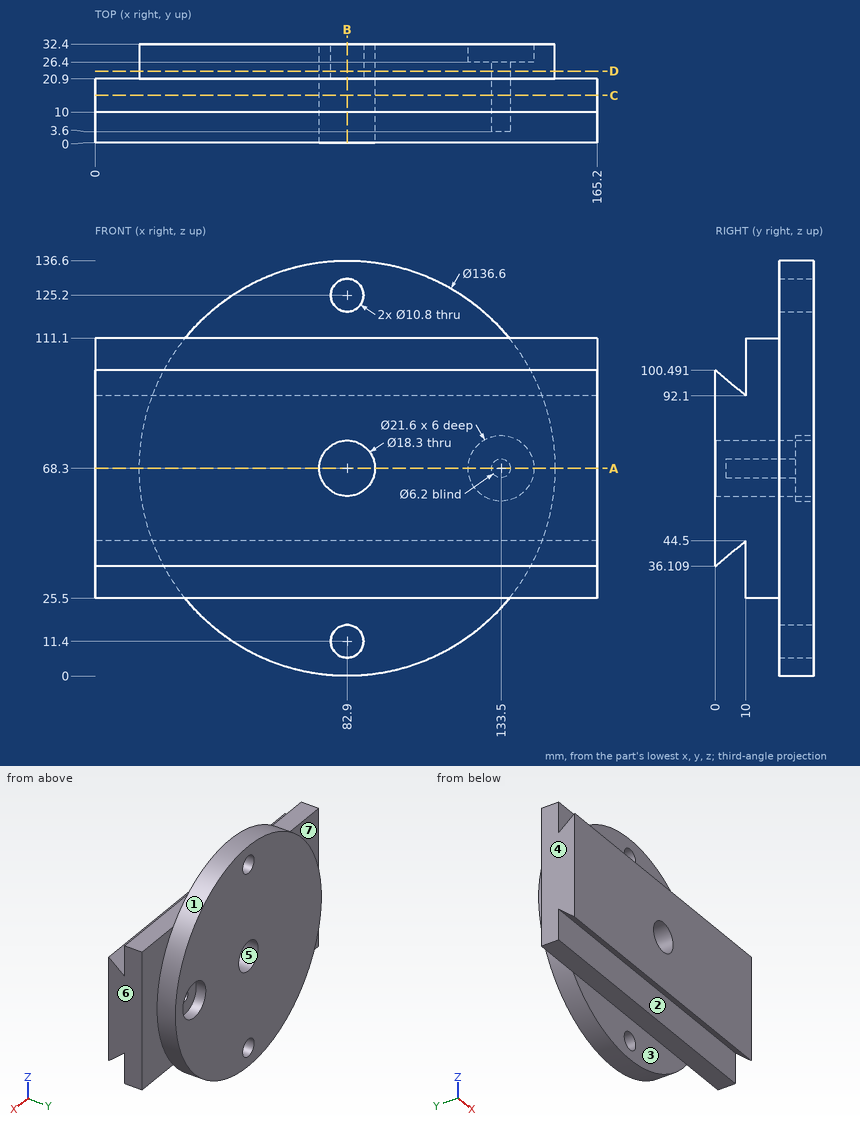
Design review of the part shown in the three views and the two pictorial views. Dimensions are in mm from the part's minimum x, y and z. A direction names the side the tool comes from. Give positions to 0.01 mm unless a question says otherwise; leave off trailing zeros. Write each loop counter-clockwise with the first axis right and the second up, starting at its lowest first coordinate (ties: lowest second). Pieces come first, ordered by that corner, then holes.
Item 1: Take a section at D-D (y = 23.5). Give the boundary of the cut face in (x, z), and give its area (3 significant figures).
Item 2: Take a section at B-B (x = 82.9). Give the boundary of the cut face in (y, z), and give its area (3 significant figures).
Item 3: Machinability: for the marked faces 1, 2 and 3, which of the approach directions +Z, -Z, +X, -X, +Y, -Y give a long, thin tool a straight path to every point of the face, cutting with its end or side? Answer none if there is none.
Item 4: Wall thickness on probe 1 along X at (y, z) = (30, 68); probe 2 along Z at (x, y) = (82.9, 28); probe 3 along Z at (x, y) = (133.5, 16.5): over which ranges is each line inside the solid? List them lowest first.
Item 5: Take a section at A-A (z = 68.3). Give the boundary of the cut face in (x, y), and give its area (3 significant figures).
Item 6: Take a section at C-C (y = 15.5). Give the boundary of the cut face in (x, z).
Item 7: Insertion check: P1, Ø20.5, axis at x = 105, z = 18, coming from the -Y side; P2, Ø1, axis at x = 50, y = 12, coming from the +Z side; P3, Ø3, axis at x = 134, z = 67.5, coming from the +Y side. Each pin has a flat end and moves straight along its axis. Give the tip position at first contact, or say it passes through.
Item 8: The part is to be moulded in two halves that separate along X. For the marked faces 4, 5, 6 and 7, say which applies: +X half, -X half, draft (parallel to the pull), parting line (faces both ways), or undercut.
Established:
1. outline: circle Ø136.6 at (82.9, 68.3); hole circle Ø18.3 at (82.9, 68.3); hole circle Ø10.8 at (82.9, 11.4); hole circle Ø10.8 at (82.9, 125.2); hole circle Ø6.2 at (133.5, 68.3)
1. area: 14,200 mm2
2. outline: (0, 36.11) - (10, 44.5) - (10, 25.5) - (20.9, 25.5) - (20.9, 16.8) - (32.4, 16.8) - (32.4, 59.15) - (0, 59.15) - close; (0, 77.45) - (32.4, 77.45) - (32.4, 119.8) - (20.9, 119.8) - (20.9, 111.1) - (10, 111.1) - (10, 92.1) - (0, 100.49) - close; (20.9, 0) - (32.4, 0) - (32.4, 6) - (20.9, 6) - close; (20.9, 130.6) - (32.4, 130.6) - (32.4, 136.6) - (20.9, 136.6) - close
2. area: 2,220 mm2
3. face 1: +Y
3. face 2: -Z, +X, -X
3. face 3: -Z, +X, -X, -Y
4. probe 1: x = 14.6 to 73.75, 92.05 to 122.7, 144.3 to 151.2
4. probe 2: z = 0 to 6, 16.8 to 59.15, 77.45 to 119.8, 130.6 to 136.6
4. probe 3: z = 25.5 to 65.2, 71.4 to 111.1
5. outline: (0, 0) - (73.75, 0) - (73.75, 32.4) - (14.6, 32.4) - (14.6, 20.9) - (0, 20.9) - close; (92.05, 0) - (165.2, 0) - (165.2, 20.9) - (151.2, 20.9) - (151.2, 32.4) - (144.3, 32.4) - (144.3, 26.4) - (136.6, 26.4) - (136.6, 3.6) - (130.4, 3.6) - (130.4, 26.4) - (122.7, 26.4) - (122.7, 32.4) - (92.05, 32.4) - close
5. area: 4,160 mm2
6. outline: (0, 25.5) - (165.2, 25.5) - (165.2, 111.1) - (0, 111.1) - close; hole circle Ø18.3 at (82.9, 68.3); hole circle Ø6.2 at (133.5, 68.3)
7. P1: stops at y = 10
7. P2: stops at z = 111.1
7. P3: stops at y = 3.6
8. face 4: -X half
8. face 5: undercut
8. face 6: +X half
8. face 7: draft
